from build123d import *

# Parameters (mm, degrees)
VALVE_BODY_START   = 15
SKETCH1_W          = 55
SKETCH1_H          = 45
VALVE_BODY_DEPTH   = 20
COIL_START         = 35
SKETCH2_W          = 35
SKETCH2_H          = 35
COIL_DEPTH         = 40
PORT_IN_G12_START  = -37.5
SKETCH3_R          = 10.45
PORT_IN_G12_DEPTH  = 10
PORT_OUT_G12_START = 27.5
SKETCH4_R          = 10.45
PORT_OUT_G12_DEPTH = 10
SKETCH5_W          = 30
SKETCH5_H          = 30
MOUNT_FOOT_DEPTH   = 15
SPADE_1_START      = 75
SKETCH6_W          = 2
SKETCH6_H          = 6
SPADE_1_DEPTH      = 6
SPADE_2_START      = 75
SKETCH7_W          = 2
SKETCH7_H          = 6
SPADE_2_DEPTH      = 6
LABEL_NC_START     = 75
LABEL_NC_DEPTH     = 0.6
FLOW_ARROW_START   = 35
FLOW_ARROW_DEPTH   = 0.6


# Read off the part's stored shape, not the designer's step: Label_NC
with BuildPart() as part:
    # Sketch1 → Valve_Body (new body)
    with BuildSketch(Plane(origin=(0, 0, 0), x_dir=(1, 0, 0), z_dir=(0, 1, 0)).offset(VALVE_BODY_START)):
        Rectangle(SKETCH1_W, SKETCH1_H)
    extrude(amount=VALVE_BODY_DEPTH)

    # Sketch2 → Coil (add)
    with BuildSketch(Plane(origin=(0, 0, 0), x_dir=(1, 0, 0), z_dir=(0, 1, 0)).offset(COIL_START)):
        Rectangle(SKETCH2_W, SKETCH2_H)
    extrude(amount=COIL_DEPTH)

    # Sketch3 → Port_In_G12 (add)
    with BuildSketch(Plane(origin=(0, 0, 0), x_dir=(0, 0, -1), z_dir=(1, 0, 0)).offset(PORT_IN_G12_START)):
        with Locations(Location((0, 25, 0), (0, 0, 253.124499321))):
            Circle(SKETCH3_R)
    extrude(amount=PORT_IN_G12_DEPTH)

    # Sketch4 → Port_Out_G12 (add)
    with BuildSketch(Plane(origin=(0, 0, 0), x_dir=(0, 0, -1), z_dir=(1, 0, 0)).offset(PORT_OUT_G12_START)):
        with Locations(Location((0, 25, 0), (0, 0, 253.124499321))):
            Circle(SKETCH4_R)
    extrude(amount=PORT_OUT_G12_DEPTH)

    # Sketch5 → Mount_Foot (add)
    with BuildSketch(Plane(origin=(0, 0, 0), x_dir=(1, 0, 0), z_dir=(0, 1, 0))):
        Rectangle(SKETCH5_W, SKETCH5_H)
    extrude(amount=MOUNT_FOOT_DEPTH)

    # Sketch6 → Spade_1 (add)
    with BuildSketch(Plane(origin=(0, 0, 0), x_dir=(1, 0, 0), z_dir=(0, 1, 0)).offset(SPADE_1_START)):
        with Locations((-6, 0)):
            Rectangle(SKETCH6_W, SKETCH6_H)
    extrude(amount=SPADE_1_DEPTH)

    # Sketch7 → Spade_2 (add)
    with BuildSketch(Plane(origin=(0, 0, 0), x_dir=(1, 0, 0), z_dir=(0, 1, 0)).offset(SPADE_2_START)):
        with Locations((6, 0)):
            Rectangle(SKETCH7_W, SKETCH7_H)
    extrude(amount=SPADE_2_DEPTH)

    # Label_NC outline → Label_NC (add)
    with BuildSketch(Plane(origin=(0, 0, 0), x_dir=(1, 0, 0), z_dir=(0, 1, 0)).offset(LABEL_NC_START)):
        with BuildLine():
            add(Edge.make_bspline(
                [(5.208984375, -7.743589744), (5.245464646, -7.744027112), (5.317673669, -7.744892838), (5.424492146, -7.753334838), (5.528489114, -7.767407896), (5.629736219, -7.786563187), (5.728726021, -7.810336972), (5.824701954, -7.8413071), (5.918227191, -7.87671881), (6.008711886, -7.917502561), (6.0957219, -7.963283105), (6.179230132, -8.013552993), (6.258573253, -8.068249902), (6.334309566, -8.12690864), (6.405172129, -8.19077019), (6.473172899, -8.258078009), (6.536002591, -8.330770835), (6.574785846, -8.381938168), (6.594230769, -8.407592147)],
                knots=[0, 0, 0, 0, 0.068547537, 0.135682946, 0.20121499, 0.265682235, 0.329266835, 0.392395428, 0.455069762, 0.51712685, 0.578790035, 0.639739863, 0.700191504, 0.759806243, 0.819628319, 0.879354791, 0.939511608, 1, 1, 1, 1], degree=3))
            add(Edge.make_bspline(
                [(3.500641026, -9.394055489), (3.502051808, -9.336945899), (3.504827435, -9.224586346), (3.528409335, -9.059691402), (3.566344958, -8.901711205), (3.620226421, -8.750940665), (3.688539133, -8.606586768), (3.772927561, -8.469752247), (3.872411326, -8.339562007), (3.98621019, -8.217991482), (4.111003416, -8.106830784), (4.244642626, -8.009035156), (4.386866249, -7.927648553), (4.536107443, -7.85961632), (4.69348374, -7.807324557), (4.858659368, -7.770718451), (5.031323955, -7.747933639), (5.149127727, -7.745053272), (5.208984375, -7.743589744)],
                knots=[0, 0, 0, 0, 0.064557846, 0.127013532, 0.18795481, 0.248013913, 0.307747682, 0.368234515, 0.429469844, 0.492743437, 0.556257769, 0.618216786, 0.679655476, 0.741245546, 0.803415265, 0.866815462, 0.932328312, 1, 1, 1, 1], degree=3))
            add(Edge.make_bspline(
                [(3.903240184, -10.526166867), (3.871094993, -10.486668788), (3.807192697, -10.408149487), (3.725435826, -10.280890061), (3.655451973, -10.148022472), (3.598868102, -10.008848679), (3.554633337, -9.863680978), (3.523988967, -9.71244619), (3.504075726, -9.555285556), (3.501798535, -9.448390755), (3.500641026, -9.394055489)],
                knots=[0, 0, 0, 0, 0.12432851, 0.247156016, 0.368779749, 0.490733862, 0.613613772, 0.738957576, 0.867310575, 1, 1, 1, 1], degree=3))
            add(Edge.make_bspline(
                [(5.212800481, -11.081410256), (5.178652297, -11.081172592), (5.111128492, -11.080702639), (5.011434625, -11.073089745), (4.914379791, -11.062703197), (4.82024138, -11.047063936), (4.728505674, -11.028608713), (4.640004287, -11.003869787), (4.553866346, -10.976157329), (4.470437923, -10.943586377), (4.389648052, -10.906832411), (4.311757309, -10.865292926), (4.236801517, -10.819317234), (4.164043742, -10.76991876), (4.094558791, -10.715510779), (4.027744522, -10.656848904), (3.963226276, -10.594130851), (3.923309554, -10.548905377), (3.903240184, -10.526166867)],
                knots=[0, 0, 0, 0, 0.069662801, 0.137749562, 0.203916744, 0.268779862, 0.332413706, 0.39475354, 0.456180032, 0.516995649, 0.577395938, 0.637198344, 0.696999184, 0.756756194, 0.816553905, 0.876947997, 0.938131788, 1, 1, 1, 1], degree=3))
            add(Edge.make_bspline(
                [(6.594230769, -10.4154998), (6.574166484, -10.441388252), (6.53413402, -10.493041154), (6.46931139, -10.565859062), (6.401024128, -10.634352008), (6.328765019, -10.697967779), (6.253365308, -10.75797933), (6.173471139, -10.812681706), (6.090132803, -10.862838436), (6.003632668, -10.908764289), (5.914062641, -10.949510649), (5.821530046, -10.98439371), (5.726433738, -11.014442717), (5.62876937, -11.039164117), (5.528334362, -11.058460028), (5.425491146, -11.071359305), (5.32001776, -11.080196613), (5.248860185, -11.081002079), (5.212800481, -11.081410256)],
                knots=[0, 0, 0, 0, 0.061674239, 0.123053062, 0.183475001, 0.243726501, 0.304278917, 0.364862921, 0.425946204, 0.48739123, 0.549220384, 0.611143589, 0.67352853, 0.736961457, 0.800785283, 0.866012596, 0.932100748, 1, 1, 1, 1], degree=3))
            Line((6.594230769, -10.4154998), (6.344911859, -10.226602564))
            add(Edge.make_bspline(
                [(5.210892428, -10.755769231), (5.266321296, -10.754237266), (5.375418567, -10.751221994), (5.535409563, -10.725677532), (5.688567722, -10.684259278), (5.834901282, -10.626294734), (5.973997711, -10.550942652), (6.106074682, -10.459595291), (6.231243678, -10.351383732), (6.306510484, -10.268758323), (6.344911859, -10.226602564)],
                knots=[0, 0, 0, 0, 0.12851519, 0.252948636, 0.374754734, 0.495939754, 0.617180641, 0.740909469, 0.867811148, 1, 1, 1, 1], degree=3))
            add(Edge.make_bspline(
                [(3.785576923, -9.415680088), (3.786721573, -9.462607785), (3.788968942, -9.554744095), (3.808969931, -9.689700291), (3.839363835, -9.818986903), (3.884916537, -9.941795759), (3.941085961, -10.059641199), (4.012061373, -10.170529301), (4.094263518, -10.276135756), (4.188855313, -10.373964716), (4.292637731, -10.463330738), (4.403987623, -10.542025909), (4.522627655, -10.607625838), (4.647247884, -10.662214018), (4.778807287, -10.704175478), (4.917069287, -10.73371579), (5.061733168, -10.752985482), (5.160583981, -10.754830328), (5.210892428, -10.755769231)],
                knots=[0, 0, 0, 0, 0.064323217, 0.126290104, 0.186726469, 0.246146432, 0.305575643, 0.365429386, 0.426326309, 0.488839906, 0.551724972, 0.613918596, 0.675483766, 0.737333897, 0.800229044, 0.864502298, 0.931040739, 1, 1, 1, 1], degree=3))
            add(Edge.make_bspline(
                [(5.191175881, -8.069230769), (5.159350317, -8.069597221), (5.095994559, -8.070326723), (5.001970587, -8.079950715), (4.909702319, -8.093477313), (4.819249775, -8.113548142), (4.730728091, -8.138923304), (4.643558555, -8.169244929), (4.559003225, -8.206759677), (4.475892395, -8.248223598), (4.39626411, -8.295057066), (4.320921317, -8.346141321), (4.250138803, -8.400904716), (4.183860577, -8.459552505), (4.122018881, -8.521820569), (4.06506182, -8.588372508), (4.013186484, -8.658995551), (3.965364611, -8.732758427), (3.922535917, -8.809446281), (3.886676669, -8.889342952), (3.854922023, -8.971080246), (3.829794853, -9.055581656), (3.809906184, -9.142252594), (3.796183232, -9.231325666), (3.78666869, -9.322614789), (3.785942816, -9.38449038), (3.785576923, -9.415680088)],
                knots=[0, 0, 0, 0, 0.043954909, 0.087501875, 0.130462627, 0.172752021, 0.215403067, 0.25764983, 0.300152749, 0.34312149, 0.385925163, 0.427685727, 0.46881795, 0.5094918, 0.549883031, 0.589980023, 0.63040523, 0.670868626, 0.711383944, 0.751627258, 0.791775577, 0.832458919, 0.873319045, 0.914542956, 0.956923558, 1, 1, 1, 1], degree=3))
            add(Edge.make_bspline(
                [(6.344911859, -8.598397436), (6.327126517, -8.577201163), (6.291795619, -8.53509439), (6.234954771, -8.475967232), (6.175716852, -8.420572316), (6.114104507, -8.368645754), (6.049008734, -8.322003402), (5.982006438, -8.278214616), (5.911976783, -8.238964596), (5.815137709, -8.191373173), (5.688457161, -8.14171059), (5.528986128, -8.100069801), (5.362515346, -8.07356202), (5.248943238, -8.070691057), (5.191175881, -8.069230769)],
                knots=[0, 0, 0, 0, 0.063163259, 0.125474941, 0.18712122, 0.248294346, 0.309294856, 0.369850066, 0.430973376, 0.49245599, 0.616147966, 0.740843698, 0.868182649, 1, 1, 1, 1], degree=3))
            Line((6.344911859, -8.598397436), (6.594230769, -8.407592147))
        make_face()
        Polygon((0.407051282, -7.825), (0.407051282, -11), (0.691987179, -11), (0.691987179, -8.506810897), (2.784485176, -11), (2.849358974, -11), (2.849358974, -7.825), (2.564423077, -7.825), (2.564423077, -10.323913261), (0.466836939, -7.825), align=None)
    extrude(amount=LABEL_NC_DEPTH)

    # Sketch9 → Flow_Arrow (add)
    with BuildSketch(Plane(origin=(0, 0, 0), x_dir=(1, 0, 0), z_dir=(0, 1, 0)).offset(FLOW_ARROW_START)):
        Polygon((-24.5, 16), (-18.5, 16), (-18.5, 19), (-13.5, 14), (-18.5, 9), (-18.5, 12), (-24.5, 12), align=None)
    extrude(amount=FLOW_ARROW_DEPTH)


solid = part.part
CAD build for the part. Positions are in the model's coordinates, mm. A direction names the side the tool comes from. Round coordinates to 2 decimals unless told otherwise and drop trailing zeros. Order: outer loops, then holes, each group sorted by start corner. A loop starts at its lowest first (then second) coordinate and runs counter-clockwise, first axis right, second up. Notation, with made-up numbers: M 49.5,-37 L 74.5,-37 A20 ccw 74.5,-22 Z; hole C -38,-40 d10. An arc over 180 degrees is marked long. Use one line per item in the form item = value.
Q1. Saw through at C-C on x = -12. Give the cut face in (y, z), then the cut area to 3 significant figures.
Recorded:
outline = M 0,-15 L 15,-15 L 15,-22.5 L 35,-22.5 L 35,-17.5 L 75,-17.5 L 75,17.5 L 35,17.5 L 35,22.5 L 15,22.5 L 15,15 L 0,15 Z
area = 2,750 mm^2
Q2. Saw through at B-B on y = 25. Give the cut face in (x, z).
Recorded:
outline = M -37.5,-10.45 L -27.5,-10.45 L -27.5,-22.5 L 27.5,-22.5 L 27.5,-10.45 L 37.5,-10.45 L 37.5,10.45 L 27.5,10.45 L 27.5,22.5 L -27.5,22.5 L -27.5,10.45 L -37.5,10.45 Z
Q3. Saw through at D-D on x = -21. Give the cut face in (y, z), then the cut area to 3 significant figures.
Recorded:
outline = M 15,-22.5 L 35,-22.5 L 35,-16 L 35.6,-16 L 35.6,-12 L 35,-12 L 35,22.5 L 15,22.5 Z
area = 902 mm^2
Q4. Flat gauge pins, fed straight in: P1, Ø3, axis at y = 78, z = -1, coming from the -X side; P2, Ø6, axis at x = 21, y = 63.5, coming from the -Z side; P3, Ø1, axis at x = -6.5, y = 79, coming from the +Z side; P4, Ø1.5, axis at x = 27, z = 10.5, coming from the +Y side. Where does each tip first touch, or does it go through?
Recorded:
P1 = -7
P2 = through
P3 = 3
P4 = 35
Q5. Two-plate mould, pull along X, no slides. Class faces 5 (the flat face through (6, 78, -3)), 6 (the flat face through (1.53, 75.3, 9.09)), 7 (the flat face through (27.5, 25, 15)), 8 (the flat face through (1.724, 75.296, 9.736)): +X half, -X half, draft (parallel to the pull), parting line (faces both ways), or undercut.
Recorded:
face_5 = draft
face_6 = undercut
face_7 = +X half
face_8 = undercut
Q6. Saw through at A-A on z = 0. Give the cut face in (x, y), then the cut area to 3 significant figures.
Recorded:
outline = M -37.5,14.55 L -27.5,14.55 L -27.5,15 L -15,15 L -15,0 L 15,0 L 15,15 L 27.5,15 L 27.5,14.55 L 37.5,14.55 L 37.5,35.45 L 27.5,35.45 L 27.5,35 L 17.5,35 L 17.5,75 L 7,75 L 7,81 L 5,81 L 5,75 L -5,75 L -5,81 L -7,81 L -7,75 L -17.5,75 L -17.5,35 L -27.5,35 L -27.5,35.45 L -37.5,35.45 Z
area = 3,390 mm^2
Q7. Which spindle directions (+Z, -Z, +X, -X, +Y, -Y) get a long thin tool onto all of the face, cutting with end or side? Do faces 1 (the flat face through (-5, 78, 0)), 2 (the flat face through (7, 78, 0)), 3 (the flat face through (6, 81, 0)), 4 (the flat face through (-6, 78, -3)). Say none if no direction does.
Recorded:
face_1 = +Z, -Z, +Y
face_2 = +Z, -Z, +X, +Y
face_3 = +Z, -Z, +X, -X, +Y
face_4 = -Z, +X, -X, +Y
Q8. Probe L1, parallel to X at y = 38, z = 11.5; L2, parallel to Y at x = 8, z = 5; L3, parallel to Y at x = -24.5, z = 18.5. List the from-to ranges inside material, lowest first.
Recorded:
L1 = -17.5 to 17.5
L2 = 0 to 75
L3 = 15 to 35
